Work out the finished part from the listing and answer in its coordinate system (mm). Give positions to 0.01 mm unless a question says otherwise; leave off trailing zeros. Order: outer loops, then holes, each group sorted by start corner. A loop starts at its lowest first (then second) coordinate and runs counter-clockwise, first axis right, second up. Notation, with made-up numbers: M -18.75,-9.75 L 22.25,-9.75 A23 ccw 22.25,26.25 Z; hole C 45.5,41.5 d2. An arc over 180 degrees is marked long. One line per item, written item: value.
from build123d import *

# Parameters (mm, degrees)
SKETCH1_R           = 1.6
SKETCH1_W           = 41.4
SKETCH1_H           = 20.5
BOSS_EXTRUDE1_DEPTH = 5


with BuildPart() as part:
    # Sketch1 → Boss-Extrude1 (new body)
    with BuildSketch(Plane.XY):
        with BuildLine():
            Line((-27.829133209, -27.087428792), (-27.829133209, -32.087428792))
            Line((-27.829133209, -32.087428792), (-12.829133209, -32.087428792))
            Line((-12.829133209, -32.087428792), (-12.829133209, -27.087428792))
            Line((-12.829133209, -27.087428792), (0.670866791, -27.087428792))
            Line((0.670866791, -27.087428792), (0.670866791, -16.087428792))
            Line((0.670866791, -16.087428792), (-0.629133209, -16.087428792))
            Line((-0.629133209, -16.087428792), (-0.629133209, -13.587428792))
            Line((-0.629133209, -13.587428792), (0.670866791, -13.587428792))
            Line((0.670866791, -13.587428792), (0.670866791, -6.587428792))
            Line((0.670866791, -6.587428792), (3.670866791, -6.587428792))
            Line((3.670866791, -6.587428792), (3.670866791, -13.587428792))
            Line((3.670866791, -13.587428792), (4.970866791, -13.587428792))
            Line((4.970866791, -13.587428792), (4.970866791, -16.087428792))
            Line((4.970866791, -16.087428792), (3.670866791, -16.087428792))
            Line((3.670866791, -16.087428792), (3.670866791, -27.087428792))
            Line((3.670866791, -27.087428792), (17.170866791, -27.087428792))
            Line((17.170866791, -27.087428792), (17.170866791, -32.087428792))
            Line((17.170866791, -32.087428792), (32.170866791, -32.087428792))
            Line((32.170866791, -32.087428792), (32.170866791, -27.087428792))
            Line((32.170866791, -27.087428792), (92.170866791, -27.087428792))
            Line((92.170866791, -27.087428792), (64.451640551, 102.268960326))
            ThreePointArc((64.451640551, 102.268960326), (59.856128602, 108.725953776), (52.005403293, 109.81112962))
            add(Edge.make_bspline(
                [(52.005403293, 109.81112962), (35.393891125, 105.212090679), (2.170866791, 100.613051738), (-31.052157544, 105.212090679), (-47.663669711, 109.81112962)],
                knots=[0.084712196, 0.084712196, 0.084712196, 0.084712196, 0.5, 0.915287804, 0.915287804, 0.915287804, 0.915287804], degree=3))
            ThreePointArc((-47.663669711, 109.81112962), (-55.51439502, 108.725953776), (-60.10990697, 102.268960326))
            Line((-60.10990697, 102.268960326), (-87.829133209, -27.087428792))
            Line((-87.829133209, -27.087428792), (-27.829133209, -27.087428792))
        make_face()
        with Locations((-9.429133209, 78.112442288)):
            Circle(SKETCH1_R, mode=Mode.SUBTRACT)
        with Locations((-9.429133209, 67.712442288)):
            Circle(SKETCH1_R, mode=Mode.SUBTRACT)
        with Locations((40.170866791, 67.712442288)):
            Circle(SKETCH1_R, mode=Mode.SUBTRACT)
        with Locations((40.170866791, 78.112442288)):
            Circle(SKETCH1_R, mode=Mode.SUBTRACT)
        with Locations((15.370866791, 72.912571208)):
            Rectangle(SKETCH1_W, SKETCH1_H, mode=Mode.SUBTRACT)
    extrude(amount=BOSS_EXTRUDE1_DEPTH)


solid = part.part
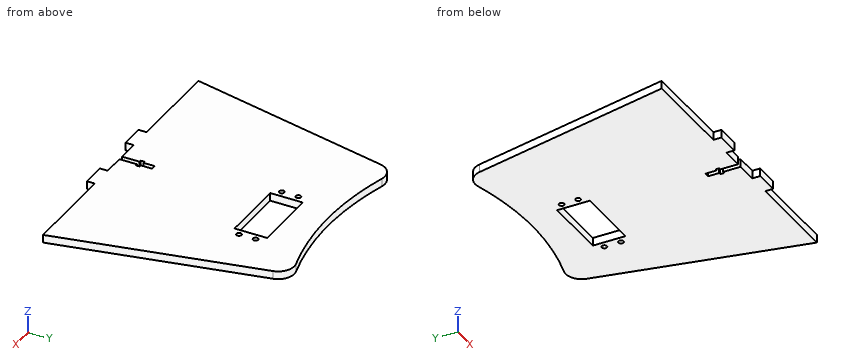
(1) Section B-B, the plane y = 26 is taken. Give the vertices of the cut face in (x, z).
Findings:
outline: M -76.45,0 L 80.79,0 L 80.79,5 L -76.45,5 Z
(2) Given P1, Ø1, axis at x = -38, z = 3, coming from the -Y side; P2, Ø1.5, axis at x = 22, z = 3.5, coming from the +Y side; P3, Ø2.5, axis at y = -23, z = 3, coming from the -X side, each flat-ended and moving along its own axis, determine where each tip first touches the part or whether it passes through.
Findings:
P1: stops at y = -27.09
P2: stops at y = 104.09
P3: stops at x = -87.22
(3) Find the intervals of material crossed by probe 1 along X at (y, z) = (-7.5, 0.8); probe 2 along Y at (x, z) = (19, 3.4); probe 3 along Y at (x, z) = (24.5, 2.25), in increasing order. Write a range as from..to.
Findings:
probe 1: x = -83.63..0.67, 3.67..87.97
probe 2: y = -32.09..62.66, 83.16..103.7
probe 3: y = -32.09..62.66, 83.16..104.3
(4) Section C-C, the plane z = 3.7 is taken. Give the number of separate pieces and of enclosed holes in the cut face, then the cut area to 4 significant figures.
Findings:
separate pieces: 1
enclosed holes: 5
area: 19,350 mm^2
(5) Section A-A, the plane x = -55 is taken. Give the vertices of the cut face in (y, z), then the cut area to 3 significant figures.
Findings:
outline: M -27.09,0 L 109.02,0 L 109.02,5 L -27.09,5 Z
area: 681 mm^2
